Verification items for the finished model (mm, model axes). Face numbers are marked on the shaded views. A direction names the side the tool comes from. Round coordinates to 2 decimals unless told otherwise and drop trailing zeros. Order: outer loops, then holes, each group sorted by start corner. A loop starts at its lowest first (then second) coordinate and runs counter-clockwise, first axis right, second up. Notation, with made-up numbers: (51.25, -35.75) -> (68.25, -35.75) arc R25 cw to (68.25, -1.75) -> close; hole circle Ø8 at (85, -35). An arc over 180 degrees is marked (long way). Put each result on its own line as item: value.
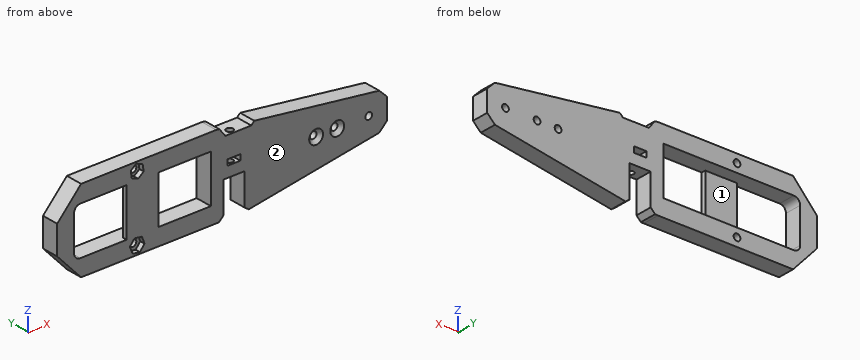
```python
from build123d import *
from OCP.BRepFilletAPI import BRepFilletAPI_MakeChamfer

# Parameters (mm, degrees)
SKETCH2_R           = 1.6
SKETCH2_W           = 6
SKETCH2_H           = 2.7
BOSS_EXTRUDE1_DEPTH = 8
SKETCH4_W           = 15
SKETCH4_H           = 38.5
BOSS_EXTRUDE2_DEPTH = 2
CHAMFER2_SIZE       = 2
CHAMFER2_SIZE2      = 2.084999334
CHAMFER2_SIZE2_2    = 1.742047362
SKETCH3_R           = 1.6
CUT_EXTRUDE1_DEPTH  = 139.590988742
CUT_EXTRUDE2_DEPTH  = 2.4
LPATTERN1_COUNT     = 2
LPATTERN1_PITCH     = 10
SKETCH7_R           = 1.6
CUT_EXTRUDE3_DEPTH  = 139.241048657
CHAMFER4_SIZE       = 4.676123657
CHAMFER4_SIZE_2     = 4
CHAMFER5_SIZE       = 1.775919651
CHAMFER5_SIZE_2     = 2


with BuildPart() as part:
    # Sketch2 → Boss-Extrude1 (new body)
    with BuildSketch(Plane(origin=(0, 0, 0), x_dir=(1, 0, 0), z_dir=(0, 1, 0))):
        Polygon((-8.652082119, -19.25), (55.5, -19.25), (61, -18.498469641), (61, -15.329705671), (71.8782498, -15.329705671), (71.8782498, -17.012045101), (133, -8.660254038), (136.660254038, -5), (136.660254038, 0), (136.660254038, 5), (133, 8.660254038), (69, 19.11), (69, 2.370294329), (59, 2.370294329), (59, 19.11), (55.5, 19.25), (-8.652082119, 19.25), (-20, 6.739512223), (-20, -6.739512223), align=None)
        with Locations(Location((18, -15.25, 0), (0, 0, 270))):
            Circle(SKETCH2_R, mode=Mode.SUBTRACT)
        with BuildLine():
            ThreePointArc((-12, 8.25), (-11.121320344, 10.371320344), (-9, 11.25))
            Line((-9, 11.25), (53, 11.25))
            Line((53, 11.25), (53, -11.25))
            Line((53, -11.25), (-9, -11.25))
            ThreePointArc((-9, -11.25), (-11.121320344, -10.371320344), (-12, -8.25))
            Line((-12, -8.25), (-12, 8.25))
        make_face(mode=Mode.SUBTRACT)
        with Locations((64, -3.979705671)):
            Rectangle(SKETCH2_W, SKETCH2_H, mode=Mode.SUBTRACT)
        with Locations(Location((128, 0, 0), (0, 0, 270))):
            Circle(SKETCH2_R, mode=Mode.SUBTRACT)
        with Locations(Location((18, 15.25, 0), (0, 0, 270))):
            Circle(SKETCH2_R, mode=Mode.SUBTRACT)
    extrude(amount=BOSS_EXTRUDE1_DEPTH)

    # Sketch4 → Boss-Extrude2 (add)
    with BuildSketch(Plane(origin=(0, 0, 0), x_dir=(-1, 0, 0), z_dir=(0, -1, 0))):
        with Locations((-20.5, 0)):
            Rectangle(SKETCH4_W, SKETCH4_H)
    extrude(amount=-BOSS_EXTRUDE2_DEPTH)

    # Chamfer2: one chamfer whose edges measure the first distance from different faces: ONE call of the kernel's chamfer builder (chamfer() names one face for all edges)
    chamfer2_edges_1 = [part.edges().sort_by_distance(p)[0] for p in [
        (59, 4, -19.11),
    ]]
    chamfer2_side_1 = [part.faces().sort_by_distance(p)[0] for p in [
        (59, 4, -10.740147164),
    ]]
    chamfer2_edges_2 = [part.edges().sort_by_distance(p)[0] for p in [
        (69, 4, -19.11),
    ]]
    chamfer2_side_2 = [part.faces().sort_by_distance(p)[0] for p in [
        (101, 4, -13.885127019),
    ]]
    chamfer2 = BRepFilletAPI_MakeChamfer(part.part.solid().wrapped)
    for e in chamfer2_edges_1:
        chamfer2.Add(CHAMFER2_SIZE, CHAMFER2_SIZE2, e.wrapped, chamfer2_side_1[0].wrapped)  # the first distance lies on this face
    for e in chamfer2_edges_2:
        chamfer2.Add(CHAMFER2_SIZE, CHAMFER2_SIZE2_2, e.wrapped, chamfer2_side_2[0].wrapped)  # the first distance lies on this face
    add(Compound.cast(chamfer2.Shape()), mode=Mode.REPLACE)

    # Sketch3 → Cut-Extrude1 (cut, through all)
    with BuildSketch(Plane(origin=(0, 0, -2.370294329), x_dir=(-1, 0, 0), z_dir=(0, 0, -1))):
        with Locations((-64, 2.5)):
            Circle(SKETCH3_R)
    extrude(amount=-CUT_EXTRUDE1_DEPTH, mode=Mode.SUBTRACT)

    # Sketch5 → Cut-Extrude2 (cut)
    with BuildSketch(Plane.XZ):
        Polygon((21.061742947, 14.043463581), (20.575762662, 17.298278962), (17.514019716, 18.504815381), (14.938257053, 16.456536419), (15.424237338, 13.201721038), (18.485980284, 11.995184619), align=None)
        Polygon((21.488981661, -15.788699565), (20.211018339, -12.49780303), (16.722036677, -11.959103466), (14.511018339, -14.711300435), (15.788981661, -18.00219697), (19.277963323, -18.540896534), align=None)
    extrude(amount=-CUT_EXTRUDE2_DEPTH, mode=Mode.SUBTRACT)

    # Sketch6 → Cut-Revolve1 (revolve, cut)
    with BuildSketch(Plane.XY, mode=Mode.PRIVATE) as cut_revolve1_sk:
        Polygon((113, 0), (113, 3.3), (109.7, 0), align=None)
    cut_revolve1 = revolve(cut_revolve1_sk.sketch.rotate(Axis((113, 0, 0), (0, 1, 0)), 270), axis=Axis((113, 0, 0), (0, 1, 0)), mode=Mode.SUBTRACT)

    # LPattern1: Cut-Revolve1 ×2
    with Locations(*[(-i * LPATTERN1_PITCH, 0, 0) for i in range(1, LPATTERN1_COUNT)]):
        add(cut_revolve1, mode=Mode.SUBTRACT)

    # Sketch7 → Cut-Extrude3 (cut, through all)
    with BuildSketch(Plane.XZ):
        with Locations(Location((113, 0, 0), (0, 0, 270))):
            Circle(SKETCH7_R)
        with Locations(Location((103, 0, 0), (0, 0, 270))):
            Circle(SKETCH7_R)
    extrude(amount=-CUT_EXTRUDE3_DEPTH, mode=Mode.SUBTRACT)

    # Chamfer4
    # the kernel refuses this chamfer: 4.676123657, 4 mm, written as the material it takes off along each edge
    with BuildSketch(Plane(origin=(61, -12.065997261, 18.498469641), x_dir=(0.023441304216062758, 0, -0.9997252148748925), z_dir=(0, 1, 0))) as chamfer4_piece_1_section:
        Polygon((CHAMFER4_SIZE * 0.999725214943, CHAMFER4_SIZE * 0.0234413042177), (-CHAMFER4_SIZE_2 * 0.158572136068, CHAMFER4_SIZE_2 * 0.98734739462), (0, 0), align=None)
    chamfer4_piece_1 = extrude(amount=32.131994523, mode=Mode.PRIVATE)
    chamfer4_piece_1 = split(chamfer4_piece_1, bisect_by=Plane(origin=(59.577955858, 4, 15.329705671), z_dir=(0, 0, 1)), keep=Keep.TOP, mode=Mode.PRIVATE)
    add(chamfer4_piece_1, mode=Mode.SUBTRACT)

    # Chamfer5
    # the kernel refuses this chamfer: 2, 1.775919651 mm, written as the material it takes off along each edge
    with BuildSketch(Plane(origin=(71.8782498, -5.143365976, 17.012045101), x_dir=(0.9949144836162346, 0, -0.10072323610091762), z_dir=(0, 1, 0))) as chamfer5_piece_1_section:
        Polygon((CHAMFER5_SIZE * 0.999390828495, CHAMFER5_SIZE * 0.0348994555423), (CHAMFER5_SIZE_2 * 0.100723236101, CHAMFER5_SIZE_2 * 0.994914483616), (0, 0), align=None)
    chamfer5_piece_1 = extrude(amount=18.286731952, mode=Mode.PRIVATE)
    chamfer5_piece_1 = split(chamfer5_piece_1, bisect_by=Plane(origin=(72.478635966, 4, 15.329705671), z_dir=(0, 0, 1)), keep=Keep.TOP, mode=Mode.PRIVATE)
    add(chamfer5_piece_1, mode=Mode.SUBTRACT)


solid = part.part
```
Item 1: Depth check by flat-ended pin: pin 1 Ø4 at (x, z) = (22.5, -3.5) entering from +Y; pin 2 Ø16.5 at (x, z) = (23.5, -5) entering from +Y; pin 3 Ø2.5 at (x, y) = (67.5, 2.5) entering from +Z; pin 4 Ø5 at (x, z) = (113, 0) entering from -Y. Enter the tip coordinate at first touch or a pass-through.
Geometry check:
pin 1: y = 2
pin 2: y = 8
pin 3: z = 15.33
pin 4: y = 0.8
Item 2: Tool access check on the marked faces 1 and 2. Record the directions out of +Z, -Z, +X, -X, +Y, -Y that give a thin tool (end or side, any length) a straight path to the whole face; none if there is none.
Geometry check:
face 1: +Y
face 2: +Z, -Z, +X, -X, -Y
Item 3: Material ranges on line 1 along Z through (x, y) = (18, 3.75); line 2 along X through (y, z) = (7.75, -5); line 3 along Z through (x, y) = (26.5, 5), recorded low to high.
Geometry check:
line 1: -19.25 to -16.85, -13.65 to -11.25, 11.25 to 13.65, 16.85 to 19.25
line 2: -20 to -12, 53 to 59, 69 to 136.66
line 3: -19.25 to -11.25, 11.25 to 19.25
Item 4: Sectioned sample at A-A, the plane x = 3. Record the boundary of the cut face in (y, z), then the cut area to 3 significant figures.
Geometry check:
outline: (0, -19.25) -> (8, -19.25) -> (8, -11.25) -> (0, -11.25) -> close; (0, 11.25) -> (8, 11.25) -> (8, 19.25) -> (0, 19.25) -> close
area: 128 mm2
Item 5: Sectioned sample at C-C, the plane x = 64. Record the boundary of the cut face in (y, z), then the cut area to 3 significant figures.
Geometry check:
outline: (0, -2.37) -> (0.9, -2.37) -> (0.9, 2.63) -> (0, 2.63) -> close; (0, 5.33) -> (0.9, 5.33) -> (0.9, 15.33) -> (0, 15.33) -> close; (4.1, -2.37) -> (8, -2.37) -> (8, 2.63) -> (4.1, 2.63) -> close; (4.1, 5.33) -> (8, 5.33) -> (8, 15.33) -> (4.1, 15.33) -> close
area: 72.0 mm2
Item 6: Sectioned sample at B-B, the plane z = 0. Give the number of separate pieces and of enclosed holes in the cut face, then the cut area to 3 significant figures.
Geometry check:
separate pieces: 6
enclosed holes: 1
area: 673 mm2
